Autodesk Inventor part; units mm, degrees
ref_plane "YZ Plane" through (0, 0, 0) normal (1, 0, 0) x (0, 1, 0)
ref_plane "XZ Plane" through (0, 0, 0) normal (0, 1, 0) x (-1, 0, 0)
ref_plane "XY Plane" through (0, 0, 0) normal (0, 0, 1) x (1, 0, 0)
sketch "Sketch1" plane through (0, 0, 0) normal (0, 0, 1) x (1, 0, 0)
  line L0 (0, 0) -> (30, 0)
  line L1 (30, 0) -> (30, 30)
  line L2 (30, 30) -> (0, 30)
  line L3 (0, 30) -> (0, 0)
  dimension "d0" = 30
  dimension "d1" = 30
extrude "Extrusion1" add sketch "Sketch1" along normal blind 12
sketch "Sketch2" plane through (0, 0, 12) normal (0, 0, 1) x (1, 0, 0)
  line L0 (30, 0) -> (30, 30)
  line L1 (30, 30) -> (0, 30)
  line L2 (0, 30) -> (0, 0)
  line L3 (0, 28) -> (30, 28)
  dimension "d7" = 2
extrude "Extrusion2" add sketch "Sketch2" along normal blind 6
pattern_linear "Rectangular Pattern1" count 8 spacing 4 along (0, -1, 0) of "Extrusion2"
sketch "Sketch3" plane through (0, 0, 0) normal (0, -1, 0) x (1, 0, 0)
  line L0 (0, 0) -> (30, 0)
  line L1 (0, 0) -> (0, 18)
  circle A0 centre (6, 6) radius 3.5
  circle A1 centre (24, 6) radius 3.5
  dimension "d11" = 18
  dimension "d12" = 7
  dimension "d13" = 6
  dimension "d14" = 6
extrude "Extrusion3" cut sketch "Sketch3" against normal blind 15
sketch "Sketch4" plane through (24, 15, 6) normal (0, -1, 0) x (1, 0, 0)
  circle A0 centre (0, 0) radius 3.5
  circle A1 centre (-18, 0) radius 3.5
  circle A2 centre (-18, 0) radius 0.925
  circle A3 centre (0, 0) radius 0.925
  point P0 (-24, -6)
  dimension "d17" = 1.85
  dimension "d18" = 1.85
extrude "Extrusion4" cut sketch "Sketch4" against normal up to next contours A2 | A3
sketch "Sketch5" plane through (0, 30, 0) normal (0, 1, 0) x (1, 0, 0)
  line L0 (30, -18) -> (0, -18)
  circle A0 centre (23.5, -15) radius 1.5
  circle A1 centre (6.5, -15) radius 1.5
  line L1 (30, 0) -> (30, -18)
  circle A2 centre (15, -3) radius 1.5
  dimension "d21" = 3
  dimension "d22" = 3
  dimension "d87" = 17
  dimension "d88" = 6.5
  dimension "d89" = 3
  dimension "d90" = 8.5
  dimension "d91" = 12
extrude "Extrusion5" cut sketch "Sketch5" against normal up to surface (2 mm away)
thread "Thread1"
thread "Thread2"
sketch "Sketch6" plane through (0, 0, 18) normal (0, 0, 1) x (1, 0, 0)
  line L0 (30, 28) -> (30, 30)
  line L1 (30, 26) -> (0, 26)
  line L2 (0, 26) -> (0, 24)
  line L3 (0, 24) -> (30, 24)
  line L4 (30, 24) -> (30, 26)
  line L5 (30, 22) -> (0, 22)
  line L6 (0, 22) -> (0, 20)
  line L7 (0, 20) -> (30, 20)
  line L8 (30, 20) -> (30, 22)
  line L9 (30, 18) -> (0, 18)
  line L10 (0, 18) -> (0, 16)
  line L11 (0, 16) -> (30, 16)
  line L12 (30, 16) -> (30, 18)
  line L13 (30, 14) -> (0, 14)
  line L14 (0, 14) -> (0, 12)
  line L15 (0, 12) -> (30, 12)
  line L16 (30, 12) -> (30, 14)
  line L17 (30, 10) -> (0, 10)
  line L18 (0, 10) -> (0, 8)
  line L19 (0, 8) -> (30, 8)
  line L20 (30, 8) -> (30, 10)
  line L21 (30, 6) -> (0, 6)
  line L22 (0, 6) -> (0, 4)
  line L23 (0, 4) -> (30, 4)
  line L24 (30, 4) -> (30, 6)
  line L25 (30, 2) -> (0, 2)
  line L26 (0, 2) -> (0, 0)
  line L27 (0, 0) -> (30, 0)
  line L28 (30, 0) -> (30, 2)
  circle A0 centre (3, 26.8635) radius 1.5
  circle A1 centre (27, 26.8635) radius 1.5
  circle A2 centre (27, 2.8635) radius 1.5
  circle A3 centre (3, 2.8635) radius 1.5
  point P0 (0, 0)
extrude "Extrusion6" cut sketch "Sketch6" against normal up to surface (6 mm away) contours A1 L1 | L1 A1 | A0 L1 | L1 A0 | A2 L25 L23 | L23 A2 | A3 L23 | L23 A3 L25 | L25 A3 | L25 A2
thread "Thread3"
thread "Thread4"
thread "Thread5"
thread "Thread6"
thread "Thread7"
thread "Thread8"
thread "Thread9"
thread "Thread10"
sketch "Sketch7" plane through (0, 30, 0) normal (0, 1, 0) x (1, 0, 0)
  circle A0 centre (24, -6) radius 0.925
  circle A1 centre (6, -6) radius 0.925
  circle A2 centre (24, -6) radius 0.925
  circle A3 centre (24, -6) radius 4
  circle A4 centre (6, -6) radius 4
  dimension "d52" = 8
extrude "Extrusion7" cut sketch "Sketch7" against normal blind 6
sketch "Sketch8" plane through (0, 0, 0) normal (0, 0, -1) x (-1, 0, 0)
  line L0 (0, 0) -> (-30, 0)
  circle A0 centre (-24, 3) radius 1.5
  circle A1 centre (-24, 11) radius 1.5
  circle A2 centre (-6, 11) radius 1.5
  circle A3 centre (-6, 3) radius 1.5
  line L1 (-20.5, 15) -> (-27.5, 15)
  line L2 (-20.5, 0) -> (-27.5, 0)
  line L3 (-2.5, 15) -> (-9.5, 15)
  line L4 (-2.5, 0) -> (-9.5, 0)
  dimension "d55" = 3
  dimension "d56" = 8
  dimension "d57" = 3.5
  dimension "d58" = 3.5
  dimension "d59" = 3
extrude "Extrusion8" cut sketch "Sketch8" against normal up to next
thread "Thread11"
thread "Thread12"
thread "Thread13"
thread "Thread14"
sketch "Sketch9" plane through (0, 0, 0) normal (0, 0, -1) x (-1, 0, 0)
  line L0 (-30, 0) -> (-30, 30)
  circle A0 centre (-15, 10) radius 1.5
  circle A1 centre (-19.5, 20) radius 1.5
  circle A2 centre (-10.5, 20) radius 1.5
  line L1 (0, 22) -> (-30, 22)
  line L2 (0, 0) -> (-30, 0)
  dimension "d70" = 3
  dimension "d73" = 10.5
  dimension "d75" = 10
  dimension "d84" = 19.5
  dimension "d85" = 15
  dimension "d86" = 20
extrude "Extrusion9" cut sketch "Sketch9" against normal blind 6
thread "Thread15"
thread "Thread16"
thread "Thread17"
properties part number "ChimeraHeatsink" material "Aluminum 6061"
For this review, take the finished solid that the model builds, in its own axes (mm). A direction names the side the tool comes from. Give positions to 0.01 mm unless a question says otherwise; leave off trailing zeros. Loops run counter-clockwise (first coordinate to the right, second up) from the corner with the lowest first, then second, coordinate; pieces in that order, holes last.
Item 1: Draft analysis for pull direction Y (two halves, no side actions). For faces 6 (the cylindrical face through (3.015, 4.363, 15.042)), 7 (the flat face through (1, 2, 15)), 8 (the flat face through (7, 24, 7)), 9 (the flat face through (30, 15, 9)), state which applies: +Y half, -Y half, draft (parallel to the pull), parting line (faces both ways), or undercut.
Item 2: Take a section at A-A, the plane y = 3. State the section outline as (x, z) points.
Item 3: Tool access review of faces 1 (the cylindrical face through (3.015, 28.363, 15.042)), 2 (the cylindrical face through (7.88, 7.4, 8.95)), 3 (the flat face through (25, 24, 7)), 4 (the cylindrical face through (25.5, 3.07, 1.4)), 5 (the flat face through (1, 4, 15)): name each direction out of +Z, -Z, +X, -X, +Y, -Y from which nothing blocks a thin tool from reaching the whole face with its end or side.
Item 4: Take a section at C-C, the plane z = 12.5. Give the number of separate pieces and of enclosed holes in the cut face, and give its area (3 significant figures).
Item 5: For line 1 along X through (y, z) = (28.95, 15); line 2 along X through (y, z) = (3, 1.75); line 3 along Y through (x, z) = (24, 2.3), list the stretches that pass through material, from the lowest coordinate up.
Item 6: Insertion check: pin 1 (1.5 mm diameter, centred on x = 26.5, z = 2, fed in from -Y); pin 2 (7 mm diameter, centred on x = 6, z = 6, fed in from +Y); pin 3 (1 mm diameter, centred on x = 9, y = 23, fed in from +Z). Each pin has a flat end and moves straight along its axis. Give the tip position at first contact, or say it passes through.
Item 7: Take a section at B-B, the plane z = 3.5. State the section outline as (x, y) points, and give its area (3 significant figures).
Item 8: Take a section at D-D, the plane z = 9. State the section outline as (x, y) points.
Calculated:
1. face 6: undercut
1. face 7: undercut
1. face 8: +Y half
1. face 9: draft
2. outline: (0, 0) - (4.5, 0) - (4.5, 2.84) arc R3.5 cw (long way) to (7.5, 2.84) - (7.5, 0) - (22.5, 0) - (22.5, 2.84) arc R3.5 cw (long way) to (25.5, 2.84) - (25.5, 0) - (30, 0) - (30, 12) - (0, 12) - close
3. face 1: +Z
3. face 2: -Y
3. face 3: +Y
3. face 4: -Z
3. face 5: +Z, +X, -X
4. separate pieces: 8
4. enclosed holes: 0
4. area: 474 mm2
5. line 1: x = 0 to 5, 8 to 22, 25 to 30
5. line 2: x = 0 to 4.5, 7.5 to 22.5, 25.5 to 30
5. line 3: y = 0 to 1.5, 4.5 to 9.5, 12.5 to 24
6. pin 1: stops at y = 0
6. pin 2: stops at y = 24
6. pin 3: stops at z = 12
7. outline: (0, 0) - (3.55, 0) - (3.55, 15) - (8.45, 15) - (8.45, 0) - (21.55, 0) - (21.55, 15) - (26.45, 15) - (26.45, 0) - (30, 0) - (30, 30) - (27.12, 30) - (27.12, 24) - (20.88, 24) - (20.88, 30) - (16.41, 30) - (16.41, 28) - (13.59, 28) - (13.59, 30) - (9.12, 30) - (9.12, 24) - (2.88, 24) - (2.88, 30) - (0, 30) - close; hole circle Ø3 at (10.5, 20); hole circle Ø3 at (15, 10); hole circle Ø3 at (19.5, 20)
7. area: 651 mm2
8. outline: (0, 0) - (4.2, 0) - (4.2, 15) - (7.8, 15) - (7.8, 0) - (22.2, 0) - (22.2, 15) - (25.8, 15) - (25.8, 0) - (30, 0) - (30, 30) - (26.65, 30) - (26.65, 24) - (21.35, 24) - (21.35, 30) - (8.65, 30) - (8.65, 24) - (3.35, 24) - (3.35, 30) - (0, 30) - close
